```python
from build123d import *

# Parameters (mm, degrees)
SKETCH1_W                = 73.58
SKETCH1_H                = 67.5
BOSS_EXTRUDE1_DEPTH      = 28
FILLET1_R                = 3
SHELL1_T                 = -2
CUT_EXTRUDE1_DEPTH       = 86.656750464
FILLET2_R                = 3
CUT_EXTRUDE3_REACH       = 162.173
CUT_EXTRUDE3_END_RADIUS  = 475
CUT_EXTRUDE3_START       = 80
FILLET3_R                = 0.3
BOSS_EXTRUDE2_REACH      = 82.024
BOSS_EXTRUDE2_END_RADIUS = 475
SKETCH5_W                = 2.5
SKETCH5_H                = 1.5
SKETCH6_W                = 14.3
SKETCH6_H                = 16.7
SKETCH6_W_2              = 11.05
SKETCH6_H_2              = 14.049996967
CUT_EXTRUDE4_DEPTH       = 2


with BuildPart() as part:
    # Sketch1 → Boss-Extrude1 (new body)
    with BuildSketch(Plane(origin=(0, 0, 0), x_dir=(1, 0, 0), z_dir=(0, 1, 0))):
        Rectangle(SKETCH1_W, SKETCH1_H)
    extrude(amount=BOSS_EXTRUDE1_DEPTH)

    # Fillet1
    fillet1_edges = [part.edges().sort_by_distance(p)[0] for p in [
        (-36.79, 28, 0),
        (36.79, 28, 0),
        (-36.79, 0, 0),
        (36.79, 0, 0),
    ]]
    fillet(fillet1_edges, radius=FILLET1_R)

    # Shell1
    shell1_openings = [part.faces().sort_by_distance(p)[0] for p in [
        (0, 14, 33.75),
    ]]
    offset(amount=SHELL1_T, openings=shell1_openings, kind=Kind.INTERSECTION)

    # Sketch2 → Cut-Extrude1 (cut, through all)
    with BuildSketch(Plane.ZY.offset(36.79)):
        with BuildLine():
            Line((18.75, 28), (33.75, 28))
            Line((33.75, 28), (33.75, 0))
            ThreePointArc((33.75, 0), (26.484121584, 14.125422277), (18.75, 28))
        make_face()
    extrude(amount=-CUT_EXTRUDE1_DEPTH, mode=Mode.SUBTRACT)

    # Fillet2
    fillet2_edges = [part.edges().sort_by_distance(p)[0] for p in [
        (0, 28, -33.75),
        (0, 0, -33.75),
        (-36.79, 14, -33.75),
        (36.79, 14, -33.75),
        (-35.911320344, 27.121320344, -33.75),
        (-35.911320344, 0.878679656, -33.75),
        (35.911320344, 0.878679656, -33.75),
        (35.911320344, 27.121320344, -33.75),
    ]]
    fillet(fillet2_edges, radius=FILLET2_R)

    # Cut-Extrude3: up to this cylinder (the profile starts outside it)
    cut_extrude3_end = Plane(origin=(0, -210.179748667, -395.218864179), z_dir=(-1, 0, 0)) * Cylinder(CUT_EXTRUDE3_END_RADIUS, 1275.346, mode=Mode.PRIVATE)
    # Sketch4 → Cut-Extrude3 (cut, up to the surface)
    with BuildSketch(Plane.XY.offset(-31.75).offset(CUT_EXTRUDE3_START), mode=Mode.PRIVATE) as cut_extrude3_sk1:
        with BuildLine():
            Line((33.79, 27), (-33.79, 27))
            ThreePointArc((-33.79, 27), (-35.204213562, 26.414213562), (-35.79, 25))
            Line((-35.79, 25), (-35.79, 3))
            ThreePointArc((-35.79, 3), (-35.204213562, 1.585786438), (-33.79, 1))
            Line((-33.79, 1), (33.79, 1))
            ThreePointArc((33.79, 1), (35.204213562, 1.585786438), (35.79, 3))
            Line((35.79, 3), (35.79, 25))
            ThreePointArc((35.79, 25), (35.204213562, 26.414213562), (33.79, 27))
        make_face()
        with BuildLine():
            Line((33.79, 26), (-33.79, 26))
            ThreePointArc((-33.79, 26), (-34.497106781, 25.707106781), (-34.79, 25))
            Line((-34.79, 25), (-34.79, 3))
            ThreePointArc((-34.79, 3), (-34.497106781, 2.292893219), (-33.79, 2))
            Line((-33.79, 2), (33.79, 2))
            ThreePointArc((33.79, 2), (34.497106781, 2.292893219), (34.79, 3))
            Line((34.79, 3), (34.79, 25))
            ThreePointArc((34.79, 25), (34.497106781, 25.707106781), (33.79, 26))
        make_face(mode=Mode.SUBTRACT)
    cut_extrude3_tool1 = extrude(cut_extrude3_sk1.sketch, amount=-CUT_EXTRUDE3_REACH, mode=Mode.PRIVATE) - cut_extrude3_end
    add(cut_extrude3_tool1.solids().sort_by_distance((0, 26.238443, 48.25))[0], mode=Mode.SUBTRACT)

    # Fillet3
    fillet3_edges = [part.edges().sort_by_distance(p)[0] for p in [
        (0, 0, 33.75),
        (-36.79, 14.077394683, 26.509847108),
        (35.984331752, 27.045704827, 19.301590008),
        (35.969562436, 0.938566613, 33.285609296),
        (-35.969562436, 0.938566613, 33.285609296),
        (-35.984331752, 27.045704827, 19.301590008),
        (36.79, 14.077394683, 26.509847108),
        (0, 28, 18.75),
    ]]
    fillet(fillet3_edges, radius=FILLET3_R)

    # Boss-Extrude2: up to this cylinder (the profile starts inside it)
    boss_extrude2_end = Plane(origin=(0, -210.179748667, -395.218864179), z_dir=(-1, 0, 0)) * Cylinder(BOSS_EXTRUDE2_END_RADIUS, 1182.128, mode=Mode.PRIVATE)
    # Sketch5 → Boss-Extrude2 (add, up to the surface)
    with BuildSketch(Plane.XY.offset(-31.75), mode=Mode.PRIVATE) as boss_extrude2_sk1:
        with Locations((33.54, 4.5)):
            Rectangle(SKETCH5_W, SKETCH5_H)
    boss_extrude2_tool1 = extrude(boss_extrude2_sk1.sketch, amount=BOSS_EXTRUDE2_REACH, mode=Mode.PRIVATE) & boss_extrude2_end
    add(boss_extrude2_tool1.solids().sort_by_distance((33.54, 4.5, -31.75))[0])
    # Sketch5 → Boss-Extrude2 (add, up to the surface)
    with BuildSketch(Plane.XY.offset(-31.75), mode=Mode.PRIVATE) as boss_extrude2_sk2:
        with Locations((33.54, 8)):
            Rectangle(SKETCH5_W, SKETCH5_H)
    boss_extrude2_tool2 = extrude(boss_extrude2_sk2.sketch, amount=BOSS_EXTRUDE2_REACH, mode=Mode.PRIVATE) & boss_extrude2_end
    add(boss_extrude2_tool2.solids().sort_by_distance((33.54, 8, -31.75))[0])
    # Sketch5 → Boss-Extrude2 (add, up to the surface)
    with BuildSketch(Plane.XY.offset(-31.75), mode=Mode.PRIVATE) as boss_extrude2_sk3:
        with Locations((-33.54, 8)):
            Rectangle(SKETCH5_W, SKETCH5_H)
    boss_extrude2_tool3 = extrude(boss_extrude2_sk3.sketch, amount=BOSS_EXTRUDE2_REACH, mode=Mode.PRIVATE) & boss_extrude2_end
    add(boss_extrude2_tool3.solids().sort_by_distance((-33.54, 8, -31.75))[0])
    # Sketch5 → Boss-Extrude2 (add, up to the surface)
    with BuildSketch(Plane.XY.offset(-31.75), mode=Mode.PRIVATE) as boss_extrude2_sk4:
        with Locations((-33.54, 4.5)):
            Rectangle(SKETCH5_W, SKETCH5_H)
    boss_extrude2_tool4 = extrude(boss_extrude2_sk4.sketch, amount=BOSS_EXTRUDE2_REACH, mode=Mode.PRIVATE) & boss_extrude2_end
    add(boss_extrude2_tool4.solids().sort_by_distance((-33.54, 4.5, -31.75))[0])

    # Sketch6 → Cut-Extrude4 (cut)
    with BuildSketch(Plane(origin=(0, 0, -33.75), x_dir=(-1, 0, 0), z_dir=(0, 0, -1))):
        with Locations((0, 10.35)):
            Rectangle(SKETCH6_W, SKETCH6_H)
        with Locations((26.425, 10.175001517)):
            Rectangle(SKETCH6_W_2, SKETCH6_H_2)
    extrude(amount=-CUT_EXTRUDE4_DEPTH, mode=Mode.SUBTRACT)


solid = part.part
```
Input: part model. Units: mm. Frame: model coordinates. A direction names the side the tool comes from. Round coordinates to 2 decimals unless told otherwise and drop trailing zeros. Loops run counter-clockwise (first coordinate to the right, second up) from the corner with the lowest first, then second, coordinate; pieces in that order, holes last. Notation, with made-up numbers: (-4, 57.5) -> (30, 57.5) arc R30 ccw to (30, 89.5) -> close; hole circle Ø2 at (56, 43). An arc over 180 degrees is marked (long way). One line per item, written item: value.
(1) Mould query, pull axis Y, two halves, no side actions, for faces 1 (the face through (7, 19, -33.75)), 2 (the face through (34, 5.25, -2)), 3 (the face through (0, 28, -6)), 4 (the face through (0, 18.7, -33)). Classes: pulls with the +Y half, pulls with the -Y half, needs draft (parallel to the pull), parting line crosses it, or undercut.
Geometry check:
face 1: needs draft
face 2: undercut
face 3: pulls with the +Y half
face 4: undercut
(2) Set-up query: faces 5 (the face through (-35.22, 1.6, 31.28)), 6 (the face through (36.79, 14, 1)), 7 (the face through (-34, 5.25, -2)), 8 (the face through (35.93, 0.9, 0.81)), 9 (the face through (-31.95, 10, -33)). Return all of +Z, -Z, +X, -X, +Y, -Y with unobstructed straight access to the full face (end or side cutting, diameter ignored); none if empty.
Geometry check:
face 5: +Z, +Y
face 6: +Z, -Z, +X, +Y, -Y
face 7: +Z
face 8: +Z, -Z, +X, -Y
face 9: +Z, -Z
(3) Section A-A (x = -1.5). Return the cut outline in (y, z), plus the area to 3 significant figures.
Geometry check:
outline: (0, -30.75) arc R3 ccw to (2, -33.58) -> (2, 29.76) arc R475 ccw to (1, 30.26) -> (1, 33.26) arc R475 ccw to (0.43, 33.54) arc R0.3 ccw to (0, 33.27) -> close; (18.7, -33.75) -> (25, -33.75) arc R3 ccw to (28, -30.75) -> (28, 18.58) arc R0.3 ccw to (27.85, 18.84) arc R475 ccw to (27, 19.33) -> (27, 16.33) arc R475 ccw to (26, 16.9) -> (26, -31.75) -> (18.7, -31.75) -> close
area: 245 mm2
(4) Section D-D (x = -29.5). Return the cut outline in (y, z).
Geometry check:
outline: (0, -30.75) arc R3 ccw to (3, -33.75) -> (3.15, -33.75) -> (3.15, -31.75) -> (2, -31.75) -> (2, 29.76) arc R475 ccw to (1, 30.26) -> (1, 33.26) arc R475 ccw to (0.43, 33.54) arc R0.3 ccw to (0, 33.27) -> close; (17.2, -33.75) -> (25, -33.75) arc R3 ccw to (28, -30.75) -> (28, 18.58) arc R0.3 ccw to (27.85, 18.84) arc R475 ccw to (27, 19.33) -> (27, 16.33) arc R475 ccw to (26, 16.9) -> (26, -31.75) -> (17.2, -31.75) -> close
(5) Material intervals for line 1 (Y direction, x = 23, z = -5); line 2 (X direction, y = 22.25, z = 13.5); line 3 (Y direction, x = 23, z = 18.5), sorted ascending. Write a range as [from, to].
Geometry check:
line 1: [0, 2], [26, 28]
line 2: [-36.79, -34.79], [34.79, 36.79]
line 3: [0, 2], [27, 28]
(6) Pin query (flat end, axial travel): pin 1 (2 mm diameter, centred on x = 23.5, y = 10.5, fed in from +Z); pin 2 (1 mm diameter, centred on x = -24.5, z = -32.5, fed in from -Y); pin 3 (10 mm diameter, centred on x = 21.5, y = 24.5, fed in from +Z). Return the tip coordinate at first contact, or that it passes through.
Geometry check:
pin 1: z = -31.75
pin 2: y = 0.27
pin 3: z = 19.33
(7) Section C-C (x = -11.5). Return the cut outline in (y, z), plus the area to 3 significant figures.
Geometry check:
outline: (0, -30.75) arc R3 ccw to (3, -33.75) -> (25, -33.75) arc R3 ccw to (28, -30.75) -> (28, 18.58) arc R0.3 ccw to (27.85, 18.84) arc R475 ccw to (27, 19.33) -> (27, 16.33) arc R475 ccw to (26, 16.9) -> (26, -31.75) -> (2, -31.75) -> (2, 29.76) arc R475 ccw to (1, 30.26) -> (1, 33.26) arc R475 ccw to (0.43, 33.54) arc R0.3 ccw to (0, 33.27) -> close
area: 278 mm2
